Geometry: see drawing. Coordinates: mm, zero at the bounding-box minimum. A direction names the side the tool comes from. Round coordinates to 2 decimals unless told otherwise and drop trailing zeros. Order: outer loops, then holes, each group sorted by start corner. A loop starts at its lowest first (then second) coordinate and runs counter-clockwise, first axis right, second up. Notation, with made-up numbers: M 83.25,3 L 107.25,3 A29 ccw 107.25,31 Z; hole C -18,32 d11. An arc over 180 degrees is marked long. Answer in a Markdown table with one row per item. Add a question column.
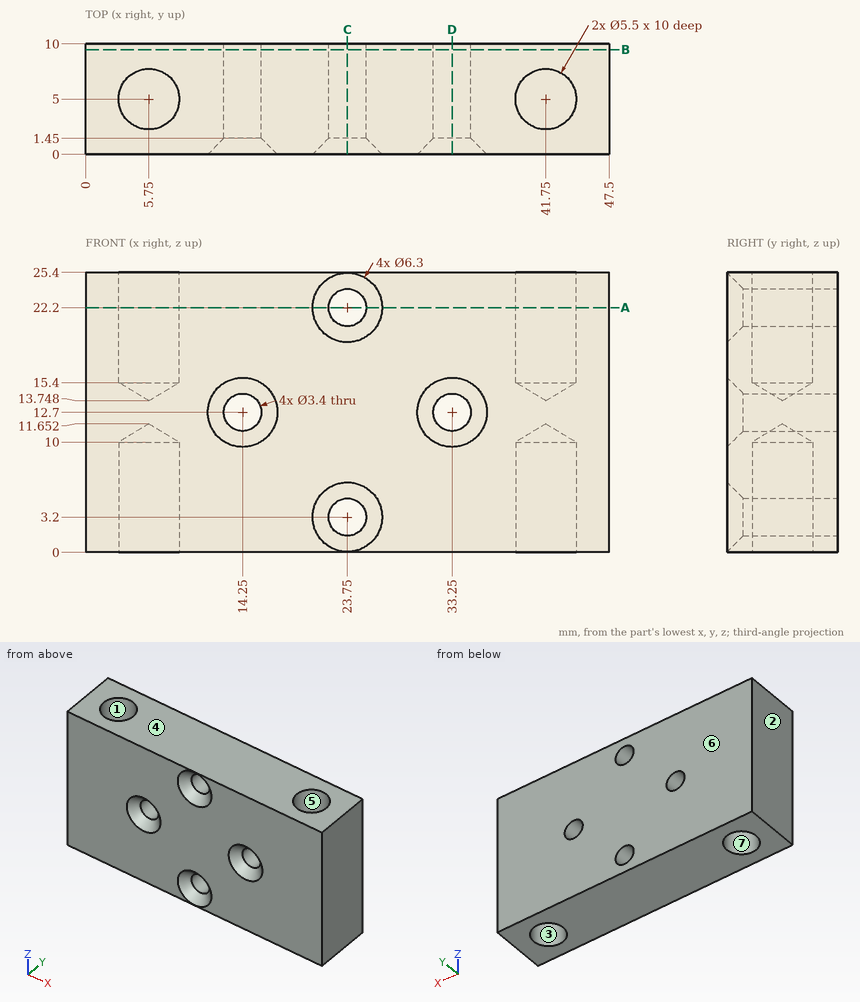
(1) Pin query (flat end, axial travel): pin 1 (5 mm diameter, centred on x = 41.75, y = 5, fed in from -Z); pin 2 (5.5 mm diameter, centred on x = 33.25, z = 12.7, fed in from -Y); pin 3 (2 mm diameter, centred on x = 14.25, z = 12.7, fed in from -Y); pin 4 (3.5 mm diameter, centred on x = 41.75, y = 5, fed in from +Z). Return the tip coordinate at first contact, or that it passes through.
(2) Access query for the marked faces 5, 6 and 7. Directions: +Z, -Z, +X, -X, +Y, -Y. A direction counts if a zero-diameter tool reaches every point of the face in a straight line with its end or side. Return the directions, or none.
(3) Cut plane D-D (x = 33.25). Return loops of the section in (y, z).
(4) Cut plane A-A (z = 22.2). Return loops of the section in (x, y).
(5) Line query: line 1 (X direction, y = 5, z = 17.5); line 2 (Y direction, x = 41.75, z = 18); line 3 (X direction, y = 3.5, z = 15.5) (1 decimal). Output: solid intervals per line, ascending. Write a range as from..to.
(6) Cut plane C-C (x = 23.75). Return loops of the section in (y, z), and give its area (3 significant figures).
(7) Draft query along X for the marked faces 1, 2, 3 and 4. Return one class per face: +X half, -X half, draft (parallel to the pull), parting line (faces both ways), or undercut.
(8) Cut plane B-B (y = 9.5). Return loops of the section in (x, z).
Answer list:
| question | item | result |
|---|---|---|
| 1 | pin 1 | z = 10.15 |
| 1 | pin 2 | y = 0.4 |
| 1 | pin 3 | through |
| 1 | pin 4 | z = 14.8 |
| 2 | face 5 | +Z |
| 2 | face 6 | +Z, -Z, +X, -X, +Y |
| 2 | face 7 | -Z |
| 3 | outline | M 0,0 L 10,0 L 10,11 L 1.45,11 L 0,9.55 Z; M 0,15.85 L 1.45,14.4 L 10,14.4 L 10,25.4 L 0,25.4 Z |
| 4 | outline | M 0,0 L 20.6,0 L 22.05,1.45 L 22.05,10 L 0,10 Z; M 25.45,1.45 L 26.9,0 L 47.5,0 L 47.5,10 L 25.45,10 Z; hole C 5.75,5 d5.5; hole C 41.75,5 d5.5 |
| 5 | line 1 | 0..3, 8.5..39, 44.5..47.5 |
| 5 | line 2 | 0..2.25, 7.75..10 |
| 5 | line 3 | 0..3.4, 8.1..39.4, 44.1..47.5 |
| 6 | outline | M 0,0 L 10,0 L 10,1.5 L 1.45,1.5 L 0,0.05 Z; M 0,6.35 L 1.45,4.9 L 10,4.9 L 10,20.5 L 1.45,20.5 L 0,19.05 Z; M 0,25.35 L 1.45,23.9 L 10,23.9 L 10,25.4 L 0,25.4 Z |
| 6 | area | 182 mm² |
| 7 | face 1 | undercut |
| 7 | face 2 | -X half |
| 7 | face 3 | undercut |
| 7 | face 4 | draft |
| 8 | outline | M 0,0 L 47.5,0 L 47.5,25.4 L 0,25.4 Z; hole C 14.25,12.7 d3.4; hole C 23.75,3.2 d3.4; hole C 23.75,22.2 d3.4; hole C 33.25,12.7 d3.4 |
